The model under review builds one solid part; all positions refer to its coordinate system, in mm. Round coordinates to 2 decimals unless told otherwise and drop trailing zeros. Write each loop counter-clockwise with the first axis right and the second up, starting at its lowest first coordinate (ties: lowest second). Pieces come first, ordered by that corner, then holes.
Item 1: Add section A-A (y = -30). Give the boundary of the cut face in (x, z).
Item 2: Add section B-B (x = 7.5). Give the boundary of the cut face in (y, z), plus the area to 3 significant figures.
Item 3: To check wall thickness, follow L1, parallel to Y at x = 7.5, z = 2.05; L2, parallel to Y at x = -6.5, z = 2.65. State the ranges of each line that lie inside material, in increasing order.
Item 4: Add section C-C (z = 2.6). Give the boundary of the cut face in (x, y).
Autodesk Inventor part; units mm, degrees
ref_plane "YZ Plane" through (0, 0, 0) normal (1, 0, 0) x (0, 1, 0)
ref_plane "XZ Plane" through (0, 0, 0) normal (0, 1, 0) x (-1, 0, 0)
ref_plane "XY Plane" through (0, 0, 0) normal (0, 0, 1) x (1, 0, 0)
sketch "Эскиз1" plane through (0, 0, 0) normal (0, 0, 1) x (1, 0, 0)
  line L0 (13.5, 5) -> (-13.5, 5)
  line L1 (-13.5, 5) -> (-13.5, -62)
  circle A0 centre (-7.5, -30) radius 1.6
  circle A1 centre (7.5, -30) radius 1.6
  circle A2 centre (7.5, -14) radius 1.6
  circle A3 centre (-7.5, -14) radius 1.6
  circle A4 centre (10, -45) radius 1.6
  circle A5 centre (1, 1) radius 1.6
  circle A6 centre (10, 1) radius 1.6
  circle A7 centre (1, -45) radius 1.6
  line L2 (13.5, 5) -> (13.5, -62)
  line L3 (13.5, -62) -> (-13.5, -62)
  circle A8 centre (4.75, -56) radius 1.1
  circle A9 centre (-4.75, -56) radius 1.1
  point P0 (0, 0)
  point P1 (13.5, -49)
extrude "Выдавливание1" add sketch "Эскиз1" along normal blind 4 contours L2 L3 L1 L0 | A4 | A5 | A6 | A7 | A8 | A9
properties part number "фанера_креп_маркера" material "Древесина (береза)"
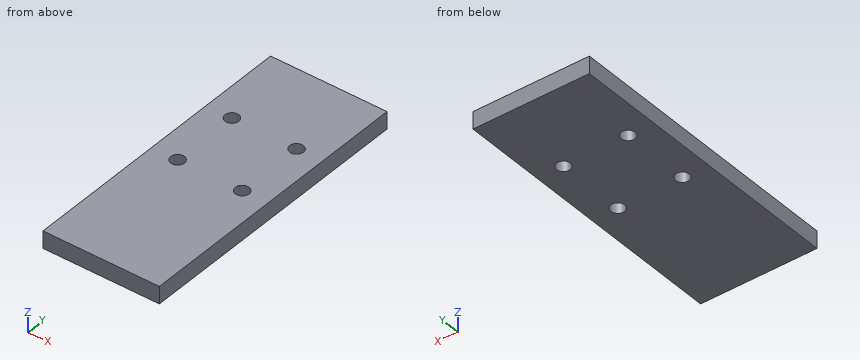
Numbers:
1. outline: (-13.5, 0) - (-9.1, 0) - (-9.1, 4) - (-13.5, 4) - close; (-5.9, 0) - (5.9, 0) - (5.9, 4) - (-5.9, 4) - close; (9.1, 0) - (13.5, 0) - (13.5, 4) - (9.1, 4) - close
2. outline: (-62, 0) - (-31.6, 0) - (-31.6, 4) - (-62, 4) - close; (-28.4, 0) - (-15.6, 0) - (-15.6, 4) - (-28.4, 4) - close; (-12.4, 0) - (5, 0) - (5, 4) - (-12.4, 4) - close
2. area: 242 mm2
3. L1: y = -62 to -31.6, -28.4 to -15.6, -12.4 to 5
3. L2: y = -62 to -31.25, -28.75 to -15.25, -12.75 to 5
4. outline: (-13.5, -62) - (13.5, -62) - (13.5, 5) - (-13.5, 5) - close; hole circle Ø3.2 at (-7.5, -30); hole circle Ø3.2 at (-7.5, -14); hole circle Ø3.2 at (7.5, -30); hole circle Ø3.2 at (7.5, -14)
